```python
from build123d import *

# Parameters (mm, degrees)
BOSS_EXTRUDE1_DEPTH           = 75
F_5_16_18_TAPPED_HOLE1_REACH  = 111.972
F_5_16_18_TAPPED_HOLE1_BORE_R = 3.2639
F_5_16_18_TAPPED_HOLE2_D      = 6.5278
SKETCH8_R                     = 2.6
CUT_EXTRUDE1_DEPTH            = 110.972346069
F_1_4_20_TAPPED_HOLE1_D       = 5.1054
F_1_4_20_TAPPED_HOLE1_DEPTH   = 13.851
FILLET1_R                     = 3.175


with BuildPart() as part:
    # Sketch1 → Boss-Extrude1 (new body)
    with BuildSketch(Plane.XY):
        Polygon((58.65, 33.52), (51.15, 41.02), (13.85, 41.02), (6.35, 33.52), (6.35, 0), (0, 0), (0, 41.02), (0, 47.37), (65, 47.37), (65, 41.02), (65, 0), (58.65, 0), align=None)
    extrude(amount=BOSS_EXTRUDE1_DEPTH)

    # 5_16-18 Tapped Hole1 bore → 5_16-18 Tapped Hole1 (cut, up to next)
    with BuildSketch(Plane.ZY, mode=Mode.PRIVATE) as f_5_16_18_tapped_hole1_sk1:
        with Locations((60, 15.87)):
            Circle(F_5_16_18_TAPPED_HOLE1_BORE_R)
    f_5_16_18_tapped_hole1_tool1 = extrude(f_5_16_18_tapped_hole1_sk1.sketch, amount=-F_5_16_18_TAPPED_HOLE1_REACH, mode=Mode.PRIVATE) & part.part
    # 5_16-18 Tapped Hole1 bore → 5_16-18 Tapped Hole1 (cut, up to next)
    with BuildSketch(Plane.ZY, mode=Mode.PRIVATE) as f_5_16_18_tapped_hole1_sk2:
        with Locations((15, 15.87)):
            Circle(F_5_16_18_TAPPED_HOLE1_BORE_R)
    f_5_16_18_tapped_hole1_tool2 = extrude(f_5_16_18_tapped_hole1_sk2.sketch, amount=-F_5_16_18_TAPPED_HOLE1_REACH, mode=Mode.PRIVATE) & part.part
    f_5_16_18_tapped_hole1_1 = f_5_16_18_tapped_hole1_tool1.solids().sort_by_distance((0, 15.87, 60))[0]
    add(f_5_16_18_tapped_hole1_1, mode=Mode.SUBTRACT)
    f_5_16_18_tapped_hole1_2 = f_5_16_18_tapped_hole1_tool2.solids().sort_by_distance((0, 15.87, 15))[0]
    add(f_5_16_18_tapped_hole1_2, mode=Mode.SUBTRACT)
    f_5_16_18_tapped_hole1 = f_5_16_18_tapped_hole1_1 + f_5_16_18_tapped_hole1_2  # 5_16-18 Tapped Hole1 as one shape, for the pattern or mirror that repeats it

    # Mirror1: 5_16-18 Tapped Hole1 across plane
    add(f_5_16_18_tapped_hole1.mirror(Plane.ZY.offset(-32.5)), mode=Mode.SUBTRACT)

    # 5_16-18 Tapped Hole2 (through all)
    with Locations(Plane(origin=(0, 47.37, 0), x_dir=(1, 0, 0), z_dir=(0, 1, 0))):
        with Locations((32.5, -15), (32.5, -60)):
            Hole(F_5_16_18_TAPPED_HOLE2_D / 2)

    # Sketch8 → Cut-Extrude1 (cut, through all)
    with BuildSketch(Plane.ZY):
        with Locations((37.5, 15.87)):
            Circle(SKETCH8_R)
    extrude(amount=-CUT_EXTRUDE1_DEPTH, mode=Mode.SUBTRACT)

    # 1_4-20 Tapped Hole1
    with Locations(Plane(origin=(0, 47.37, 0), x_dir=(1, 0, 0), z_dir=(0, 1, 0))):
        with Locations((54.9, -57.5), (54.9, -37.5), (54.9, -17.5)):
            f_1_4_20_tapped_hole1 = Hole(F_1_4_20_TAPPED_HOLE1_D / 2, depth=F_1_4_20_TAPPED_HOLE1_DEPTH)

    # Mirror2: 1_4-20 Tapped Hole1 across plane
    add(f_1_4_20_tapped_hole1.mirror(Plane.ZY.offset(-32.5)), mode=Mode.SUBTRACT)

    # Fillet1
    fillet1_edges = [part.edges().sort_by_distance(p)[0] for p in [
        (58.65, 0, 37.5),
        (65, 0, 37.5),
        (0, 0, 37.5),
        (6.35, 0, 37.5),
        (0, 47.37, 37.5),
        (65, 47.37, 37.5),
    ]]
    fillet(fillet1_edges, radius=FILLET1_R - 0.0001)  # a hair under: the kernel refuses the full size


solid = part.part
```
Here's how the part is built. I have some questions about the finished solid (model axes, mm). A direction names the side the tool comes from. Round coordinates to 2 decimals unless told otherwise and drop trailing zeros. Order: outer loops, then holes, each group sorted by start corner. A loop starts at its lowest first (then second) coordinate and runs counter-clockwise, first axis right, second up. Notation, with made-up numbers: (87.25, 20.5) -> (103.25, 20.5) arc R19 ccw to (103.25, 44.5) -> close; hole circle Ø4 at (89.25, -17.5). An arc over 180 degrees is marked (long way). Use a Markdown table: item, result. Add a question column.
(1) For faces 4 (the face through (57.45, 42.32, 57.39)), 5 (the face through (5.44, 0.95, 38.02)), which set-ups out of +Z, -Z, +X, -X, +Y, -Y let a thin tool reach every point of the face, with its end or its side?
(2) Suppose I cut it at B-B, the plane x = 32.5. Please give me the cut outline in (y, z).
(3) Suppose I cut it at D-D, the plane x = 54.9. Please give me the cut outline in (y, z), and give its area (3 significant figures).
(4) Suppose I cut it at C-C, the plane z = 37.5. Count the separate pieces of the cut face and the enclosed holes in it, and give its area (3 significant figures).
(5) I need wall thicknesses on line 1 along Z through (x, y) = (54.9, 37.75); line 2 along X through (y, z) = (32, 30.5). Which ranges of each line are inside material? Lowest first, please.
(6) Suppose I cut it at A-A, the plane y = 23. Please give me the cut outline in (x, z).
(7) If we mould it in two halves opening along X, with no side actions, what happens to faces 1 (the face through (61.869, 16.85, 63.113)), 2 (the face through (0.95, 0.91, 38.02)), 3 (the face through (58.29, 33.88, 36.98))? For each: released by +X, released by -X, zero draft, split by the parting line, or undercut.
(8) For pin 1 Ø8.5 at (y, z) = (15.87, 37.5) entering from -X; pin 2 Ø4.5 at (x, z) = (10.1, 37.5) entering from -Y; pin 3 Ø12 at (x, z) = (26, 35.5) entering from -Y; pin 4 Ø6 at (x, z) = (10.1, 57.5) entering from -Y, each with a flat end and sliding along its axis, tell me the tip position at first contact or that it passes through.
Verdict:
| question | item | result |
|---|---|---|
| 1 | face 4 | +Y, -Y |
| 1 | face 5 | +Z, -Z, -Y |
| 2 | outline | (41.02, 0) -> (47.37, 0) -> (47.37, 11.74) -> (41.02, 11.74) -> close; (41.02, 18.26) -> (47.37, 18.26) -> (47.37, 56.74) -> (41.02, 56.74) -> close; (41.02, 63.26) -> (47.37, 63.26) -> (47.37, 75) -> (41.02, 75) -> close |
| 3 | outline | (37.27, 0) -> (47.37, 0) -> (47.37, 14.95) -> (37.27, 14.95) -> close; (37.27, 20.05) -> (47.37, 20.05) -> (47.37, 34.95) -> (37.27, 34.95) -> close; (37.27, 40.05) -> (47.37, 40.05) -> (47.37, 54.95) -> (37.27, 54.95) -> close; (37.27, 60.05) -> (47.37, 60.05) -> (47.37, 75) -> (37.27, 75) -> close |
| 3 | area | 603 mm2 |
| 4 | separate pieces | 5 |
| 4 | enclosed holes | 0 |
| 4 | area | 808 mm2 |
| 5 | line 1 | 0 to 14.95, 20.05 to 34.95, 40.05 to 54.95, 60.05 to 75 |
| 5 | line 2 | 0 to 6.35, 58.65 to 65 |
| 6 | outline | (0, 0) -> (6.35, 0) -> (6.35, 75) -> (0, 75) -> close; (58.65, 0) -> (65, 0) -> (65, 75) -> (58.65, 75) -> close |
| 7 | face 1 | zero draft |
| 7 | face 2 | released by -X |
| 7 | face 3 | undercut |
| 8 | pin 1 | x = 0 |
| 8 | pin 2 | through |
| 8 | pin 3 | y = 41.02 |
| 8 | pin 4 | y = 34.27 |
